```python
from build123d import *

# Parameters (mm, degrees)
SKETCH1_W           = 40
SKETCH1_H           = 40
BOSS_EXTRUDE1_DEPTH = 18
SKETCH2_R           = 1.7
CUT_EXTRUDE1_DEPTH  = 34.526109228
SKETCH3_W           = 36
SKETCH3_H           = 20
CUT_EXTRUDE2_DEPTH  = 16
CIRPATTERN1_COUNT   = 2
CIRPATTERN1_ANGLE   = 90
FILLET1_R           = 4


with BuildPart() as part:
    # Sketch1 → Boss-Extrude1 (new body)
    with BuildSketch(Plane(origin=(0, 0, 0), x_dir=(1, 0, 0), z_dir=(0, 1, 0))):
        Rectangle(SKETCH1_W, SKETCH1_H)
    extrude(amount=BOSS_EXTRUDE1_DEPTH)

    # Sketch2 → Cut-Extrude1 (cut, through all)
    with BuildSketch(Plane(origin=(0, 18, 0), x_dir=(1, 0, 0), z_dir=(0, 1, 0))):
        with Locations(Location((15, 15, 0), (0, 0, 270))):
            Circle(SKETCH2_R)
        with Locations(Location((15, -15, 0), (0, 0, 270))):
            Circle(SKETCH2_R)
        with Locations(Location((-15, -15, 0), (0, 0, 270))):
            Circle(SKETCH2_R)
        with Locations(Location((-15, 15, 0), (0, 0, 270))):
            Circle(SKETCH2_R)
    extrude(amount=-CUT_EXTRUDE1_DEPTH, mode=Mode.SUBTRACT)

    # Sketch3 → Cut-Extrude2 (cut)
    with BuildSketch(Plane(origin=(0, 18, 0), x_dir=(1, 0, 0), z_dir=(0, 1, 0))):
        Rectangle(SKETCH3_W, SKETCH3_H)
    cut_extrude2 = extrude(amount=-CUT_EXTRUDE2_DEPTH, mode=Mode.SUBTRACT)

    # CirPattern1: Cut-Extrude2 ×2 about axis
    cirpattern1_axis = Axis((0, 0, 0), (0, -1, 0))
    for i in range(1, CIRPATTERN1_COUNT):
        add(cut_extrude2.rotate(cirpattern1_axis, i * CIRPATTERN1_ANGLE / (CIRPATTERN1_COUNT - 1)), mode=Mode.SUBTRACT)

    # Fillet1
    fillet1_edges = [part.edges().sort_by_distance(p)[0] for p in [
        (20, 9, -20),
        (-20, 9, -20),
        (-20, 9, 20),
        (20, 9, 20),
        (-10, 10, 18),
        (-10, 10, 10),
        (-18, 10, 10),
        (-18, 10, -10),
        (-10, 10, -10),
        (-10, 10, -18),
        (10, 10, -18),
        (10, 10, -10),
        (18, 10, -10),
        (18, 10, 10),
        (10, 10, 18),
        (10, 10, 10),
    ]]
    fillet(fillet1_edges, radius=FILLET1_R - 0.0001)  # a hair under: the kernel refuses the full size


solid = part.part
```
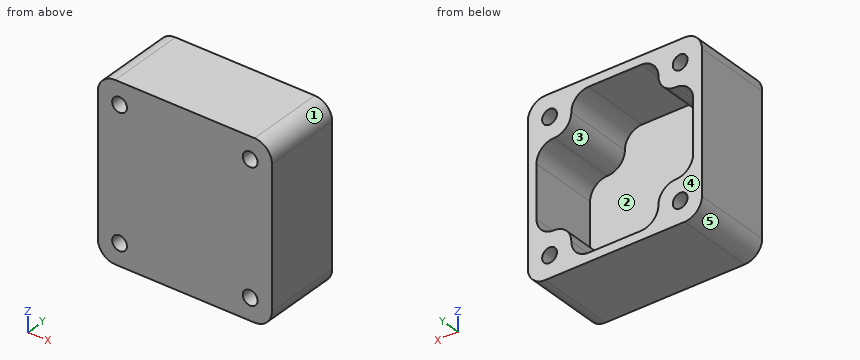
Work out the finished part from the listing and answer in its coordinate system (mm). Face numbers are marked on the shaded views. A direction names the side the tool comes from. Round coordinates to 2 decimals unless told otherwise and drop trailing zeros. Write each loop counter-clockwise with the first axis right and the second up, starting at its lowest first coordinate (ties: lowest second). Pieces come first, ordered by that corner, then holes. Notation, with made-up numbers: (4, 89.5) -> (30, 89.5) arc R18 ccw to (30, 94.5) -> close; hole circle Ø2 at (-12.5, -0.75). An arc over 180 degrees is marked (long way). Write each question's results on one line, items separated by ' | '.
Q1. Which of the six approach directions +Z, -Z, +X, -X, +Y, -Y give full straight-line access (tool end or side, diameter ignored) to the marked faces 1 and 2?
Data:
face 1: +Z, +X, +Y, -Y | face 2: +Y
Q2. Section D-D, the plane x = -15 is taken. Write down the section's boundary in (y, z).
Data:
outline: (0, -20) -> (18, -20) -> (18, -16.7) -> (0, -16.7) -> close; (0, -13.3) -> (18, -13.3) -> (18, -9.87) -> (2, -9.87) -> (2, 9.87) -> (18, 9.87) -> (18, 13.3) -> (0, 13.3) -> close; (0, 16.7) -> (18, 16.7) -> (18, 20) -> (0, 20) -> close
Q3. Straight lines are drawn through the part: line 1 along Z through (x, y) = (1, 5.75); line 2 along X through (y, z) = (5.75, -13.5). For each, find the intervals that lie inside material, in ascending order. Write a range as [from, to].
Data:
line 1: [-20, -18], [18, 20] | line 2: [-20, -15.8], [-14.2, -10.03], [10.03, 14.2], [15.8, 20]
Q4. Determine the mould class of the marked faces 3, 4 and 5 for opening direction X: released by +X, released by -X, zero draft, split by the parting line, or undercut.
Data:
face 3: undercut | face 4: zero draft | face 5: released by -X
Q5. Section B-B, the plane z = 15 is taken. Write down the section's boundary in (x, y).
Data:
outline: (-20, 0) -> (-16.7, 0) -> (-16.7, 18) -> (-20, 18) -> close; (-13.3, 0) -> (13.3, 0) -> (13.3, 18) -> (9.87, 18) -> (9.87, 2) -> (-9.87, 2) -> (-9.87, 18) -> (-13.3, 18) -> close; (16.7, 0) -> (20, 0) -> (20, 18) -> (16.7, 18) -> close
Q6. Section C-C, the plane z = -10.5 is taken. Write down the section's boundary in (x, y), then the cut area to 3 significant figures.
Data:
outline: (-20, 0) -> (20, 0) -> (20, 18) -> (12.06, 18) -> (12.06, 2) -> (-12.06, 2) -> (-12.06, 18) -> (-20, 18) -> close | area: 334 mm^2
Q7. A flat-ended cylindrical pin translates along its axis: P1, Ø11, axis at x = -4, z = -5, coming from the +Y side. Find the tip coordinate at first contact, or state that the pin passes through.
Data:
P1: y = 2
Q8. Section A-A, the plane x = 0.5 is taken. Write down the section's boundary in (y, z).
Data:
outline: (0, -20) -> (18, -20) -> (18, -18) -> (2, -18) -> (2, 18) -> (18, 18) -> (18, 20) -> (0, 20) -> close
